Could you check a few things on this model? Use its own coordinates, in mm. A direction names the side the tool comes from. Give positions to 0.01 mm unless a question says otherwise; leave off trailing zeros. Loops run counter-clockwise (first coordinate to the right, second up) from the corner with the lowest first, then second, coordinate; pieces in that order, holes last. Notation, with made-up numbers: M 79.25,29.5 L 101.25,29.5 A31 ccw 101.25,62.5 Z; hole C 19.25,28.25 d6. An arc over 180 degrees is marked long. Answer in a Markdown table with one row per item. Add a question column.
1. If we section it at A-A on z = 0: Count the separate pieces of the cut face and the enclosed holes in it, then the cut area to 3 significant figures.
2. Thinking about a two-plate mould opening in Y: for faces 4 (the flat face through (-3, 0, 3)), 5 (the flat face through (0, -5, 2)), 6 (the cylindrical face through (-3.24, -4.42, 1.27)), 7 (the cylindrical face through (-4.461, 15.735, 0.228)), which applies, released by +Y, released by -Y, zero draft, split by the parting line, or undercut?
3. Which directions (+Z, -Z, +X, -X, +Y, -Y) give clear straight access to the entire face, cutting with the end or side of a thin tool? Please do faces 1 (the flat face through (0, -5, -2)), 2 (the flat face through (1.5, 16, 0)), 3 (the flat face through (0, -8, -3)).
4. I'm going to push flat-ended pins straight in: pin 1 Ø2.5 at (x, y) = (0.5, -5.5) entering from -Z; pin 2 Ø1.2 at (x, z) = (-1, -0.5) entering from -Y; pin 3 Ø3 at (y, z) = (-6, -1) entering from -X; pin 4 Ø3 at (y, z) = (-3.45, 0) entering from -X. Where does each tip first touch, or does it pass through?
5. If we section it at D-D on x = 0.75: List the corners of the cut face in (y, z) for me, then the cut area to 3 significant figures.
6. If we section it at B-B on x = 3: List the corners of the cut face in (y, z) for me, then the cut area to 3 significant figures.
7. I need wall thicknesses on line 1 along Y through (x, z) = (5.75, 0); line 2 along X through (y, z) = (12, -3.75); line 3 along Y through (x, z) = (-0.5, -2.5). Which ranges of each line are inside material? Lowest first, please. Write a range as from..to.
8. If we section it at C-C on z = -4.5: List the corners of the cut face in (x, y) for me.
```python
from build123d import *

# Parameters (mm, degrees)
SKETCH1_R           = 7.5
BOSS_EXTRUDE1_DEPTH = 20
SKETCH2_W           = 3
SKETCH2_H           = 13
CUT_EXTRUDE1_DEPTH  = 10
SKETCH3_R           = 1.75
CUT_EXTRUDE2_DEPTH  = 27.100766272
SKETCH4_R           = 4
BOSS_EXTRUDE2_DEPTH = 8
SKETCH5_W           = 5
SKETCH5_H           = 4
CUT_EXTRUDE3_DEPTH  = 6.2
SKETCH6_R           = 1.6
CUT_EXTRUDE4_DEPTH  = 27.100766436


with BuildPart() as part:
    # Sketch1 → Boss-Extrude1 (new body)
    with BuildSketch(Plane(origin=(0, 0, 0), x_dir=(1, 0, 0), z_dir=(0, 1, 0))):
        with Locations(Location((0, 0, 0), (0, 0, 270))):
            Circle(SKETCH1_R)
    extrude(amount=BOSS_EXTRUDE1_DEPTH)

    # Sketch2 → Cut-Extrude1 (cut)
    with BuildSketch(Plane(origin=(0, 20, 0), x_dir=(1, 0, 0), z_dir=(0, 1, 0))):
        Rectangle(SKETCH2_W, SKETCH2_H)
    extrude(amount=-CUT_EXTRUDE1_DEPTH, mode=Mode.SUBTRACT)

    # Sketch3 → Cut-Extrude2 (cut, through all)
    with BuildSketch(Plane(origin=(7.5, 0, 0), x_dir=(0, 0, -1), z_dir=(1, 0, 0))):
        with Locations((0, 14)):
            Circle(SKETCH3_R)
    extrude(amount=-CUT_EXTRUDE2_DEPTH, mode=Mode.SUBTRACT)

    # Sketch4 → Boss-Extrude2 (add)
    with BuildSketch(Plane.XZ):
        with Locations(Location((0, 0, 0), (0, 0, 270))):
            Circle(SKETCH4_R)
    extrude(amount=BOSS_EXTRUDE2_DEPTH)

    # Sketch5 → Cut-Extrude3 (cut)
    with BuildSketch(Plane.XZ.offset(8)):
        Rectangle(SKETCH5_W, SKETCH5_H)
    extrude(amount=-CUT_EXTRUDE3_DEPTH, mode=Mode.SUBTRACT)

    # Sketch6 → Cut-Extrude4 (cut, through all)
    with BuildSketch(Plane(origin=(7.5, 0, 0), x_dir=(0, 0, -1), z_dir=(1, 0, 0))):
        with Locations((0, -3.45)):
            Circle(SKETCH6_R)
    extrude(amount=-CUT_EXTRUDE4_DEPTH, mode=Mode.SUBTRACT)


solid = part.part
```
Results:
| question | item | result |
|---|---|---|
| 1 | separate pieces | 5 |
| 1 | enclosed holes | 0 |
| 1 | area | 251 mm2 |
| 2 | face 4 | released by -Y |
| 2 | face 5 | zero draft |
| 2 | face 6 | undercut |
| 2 | face 7 | undercut |
| 3 | face 1 | -Y |
| 3 | face 2 | +Y |
| 3 | face 3 | +Z, -Z, +X, -X, -Y |
| 4 | pin 1 | z = -4 |
| 4 | pin 2 | y = -1.8 |
| 4 | pin 3 | x = -4 |
| 4 | pin 4 | through |
| 5 | outline | M -8,-3.93 L 0,-3.93 L 0,-7.46 L 20,-7.46 L 20,-6.5 L 10,-6.5 L 10,6.5 L 20,6.5 L 20,7.46 L 0,7.46 L 0,3.93 L -8,3.93 L -8,2 L -1.8,2 L -1.8,-2 L -8,-2 Z |
| 5 | area | 207 mm2 |
| 6 | outline | M -8,-2.65 L 0,-2.65 L 0,-6.87 L 20,-6.87 L 20,6.87 L 0,6.87 L 0,2.65 L -8,2.65 Z; hole C -3.45,0 d3.2; hole C 14,0 d3.5 |
| 6 | area | 300 mm2 |
| 7 | line 1 | 0..12.25, 15.75..20 |
| 7 | line 2 | -6.5..-1.5, 1.5..6.5 |
| 7 | line 3 | -8..10 |
| 8 | outline | M -6,0 L 6,0 L 6,20 L 1.5,20 L 1.5,10 L -1.5,10 L -1.5,20 L -6,20 Z |
